```python
from build123d import *

# Parameters (mm, degrees)
CROQUIS1_R              = 1.25
SALIENTE_EXTRUIR3_DEPTH = 3
CROQUIS7_W              = 0.5
CROQUIS7_H              = 4.35
SALIENTE_EXTRUIR4_DEPTH = 1.5
CROQUIS8_R              = 0.75
CORTAR_EXTRUIR1_DEPTH   = 21.944510021
SALIENTE_EXTRUIR5_DEPTH = 1.5
CROQUIS10_R             = 0.5
SALIENTE_EXTRUIR6_DEPTH = 2
CORTAR_EXTRUIR2_REACH   = 27.447
CROQUIS11_W             = 3.6
CROQUIS11_H             = 5.5
CROQUIS12_R             = 2.25
SALIENTE_EXTRUIR8_DEPTH = 3.6
CROQUIS13_R             = 1
SALIENTE_EXTRUIR9_DEPTH = 2.1


with BuildPart() as part:
    # Croquis1 → Saliente-Extruir3 (new, symmetric)
    with BuildSketch(Plane.XY):
        with BuildLine():
            Line((-9.25, 5), (-3.39, 5))
            ThreePointArc((-3.39, 5), (-3.319289322, 4.970710678), (-3.29, 4.9))
            Line((-3.29, 4.9), (-3.29, 4.8))
            ThreePointArc((-3.29, 4.8), (-3.202132034, 4.587867966), (-2.99, 4.5))
            Line((-2.99, 4.5), (9.25, 4.5))
            ThreePointArc((9.25, 4.5), (9.780330086, 4.280330086), (10, 3.75))
            Line((10, 3.75), (10, -4.25))
            ThreePointArc((10, -4.25), (9.780330086, -4.780330086), (9.25, -5))
            Line((9.25, -5), (-9.25, -5))
            ThreePointArc((-9.25, -5), (-9.780330086, -4.780330086), (-10, -4.25))
            Line((-10, -4.25), (-10, 4.25))
            ThreePointArc((-10, 4.25), (-9.780330086, 4.780330086), (-9.25, 5))
        make_face()
        with Locations((-4.5, -2.5)):
            Circle(CROQUIS1_R, mode=Mode.SUBTRACT)
        with Locations((5, -2.5)):
            Circle(CROQUIS1_R, mode=Mode.SUBTRACT)
    extrude(amount=SALIENTE_EXTRUIR3_DEPTH, both=True)

    # Croquis7 → Saliente-Extruir4 (add, symmetric)
    with BuildSketch(Plane.XY):
        with Locations((-8.05, -7.175)):
            Rectangle(CROQUIS7_W, CROQUIS7_H)
        with Locations((0.95, -7.175)):
            Rectangle(CROQUIS7_W, CROQUIS7_H)
        with Locations((8.25, -7.175)):
            Rectangle(CROQUIS7_W, CROQUIS7_H)
    extrude(amount=SALIENTE_EXTRUIR4_DEPTH, both=True)

    # Croquis8 → Cortar-Extruir1 (cut, through all)
    with BuildSketch(Plane(origin=(8.5, 0, 0), x_dir=(0, 0, -1), z_dir=(1, 0, 0))):
        with Locations((0, -7.85)):
            Circle(CROQUIS8_R)
        Polygon((-1.5, -9.152010101), (-1.5, -9.35), (-1.302010101, -9.35), align=None)
        Polygon((1.302010101, -9.35), (1.5, -9.152010101), (1.5, -9.35), align=None)
    extrude(amount=-CORTAR_EXTRUIR1_DEPTH, mode=Mode.SUBTRACT)

    # Croquis9 → Saliente-Extruir5 (add, symmetric)
    with BuildSketch(Plane.XY):
        with BuildLine():
            Line((-1.48, 4.5), (0.52, 4.5))
            Line((0.52, 4.5), (0.52, 6.15))
            ThreePointArc((0.52, 6.15), (0.490710678, 6.220710678), (0.42, 6.25))
            Line((0.42, 6.25), (-1.38, 6.25))
            ThreePointArc((-1.38, 6.25), (-1.450710678, 6.220710678), (-1.48, 6.15))
            Line((-1.48, 6.15), (-1.48, 4.5))
        make_face()
    extrude(amount=SALIENTE_EXTRUIR5_DEPTH, both=True)

    # Croquis10 → Saliente-Extruir6 (add, symmetric)
    with BuildSketch(Plane.XY):
        with BuildLine():
            Line((-6.45, 5), (-6.24, 5))
            ThreePointArc((-6.24, 5), (-6.120788655, 5.324037035), (-5.82, 5.493558507))
            Line((-5.82, 5.493558507), (11.429810709, 8.44212265))
            Line((11.429810709, 8.44212265), (10.840097881, 11.892084791))
            ThreePointArc((10.840097881, 11.892084791), (8.877970038, 13.281348744), (7.488706086, 11.319220901))
            Line((7.488706086, 11.319220901), (8.044721038, 8.066399453))
            Line((8.044721038, 8.066399453), (-6.05083857, 5.657001325))
            ThreePointArc((-6.05083857, 5.657001325), (-6.380057775, 5.449678442), (-6.460998376, 5.06913057))
            Line((-6.460998376, 5.06913057), (-6.45, 5))
        make_face()
        with Locations((9.164401983, 11.605652846)):
            Circle(CROQUIS10_R, mode=Mode.SUBTRACT)
    extrude(amount=SALIENTE_EXTRUIR6_DEPTH, both=True)

    # Croquis11 → Cortar-Extruir2 (cut, up to next)
    with BuildSketch(Plane(origin=(12.50740608, 2.137930074, 0), x_dir=(0, 0, -1), z_dir=(0.9857034690888546, 0.16848937956499643, 0)), mode=Mode.PRIVATE) as cortar_extruir2_sk1:
        with Locations((0, 9.345627867)):
            Rectangle(CROQUIS11_W, CROQUIS11_H)
    cortar_extruir2_tool1 = extrude(cortar_extruir2_sk1.sketch, amount=-CORTAR_EXTRUIR2_REACH, mode=Mode.PRIVATE) & part.part
    add(cortar_extruir2_tool1.solids().sort_by_distance((10.932767, 11.349948, 0))[0], mode=Mode.SUBTRACT)

    # Croquis12 → Saliente-Extruir8 (add)
    with BuildSketch(Plane(origin=(0, 0, 1.8), x_dir=(-1, 0, 0), z_dir=(0, 0, -1))):
        with Locations(Location((-9.164401983, 11.605652846, 0), (0, 0, 211.22606331))):
            Circle(CROQUIS12_R)
    extrude(amount=SALIENTE_EXTRUIR8_DEPTH)

    # Croquis13 → Saliente-Extruir9 (add, symmetric)
    with BuildSketch(Plane.XY):
        with Locations((9.164401983, 11.605652846)):
            Circle(CROQUIS13_R)
    extrude(amount=SALIENTE_EXTRUIR9_DEPTH, both=True)


solid = part.part
```
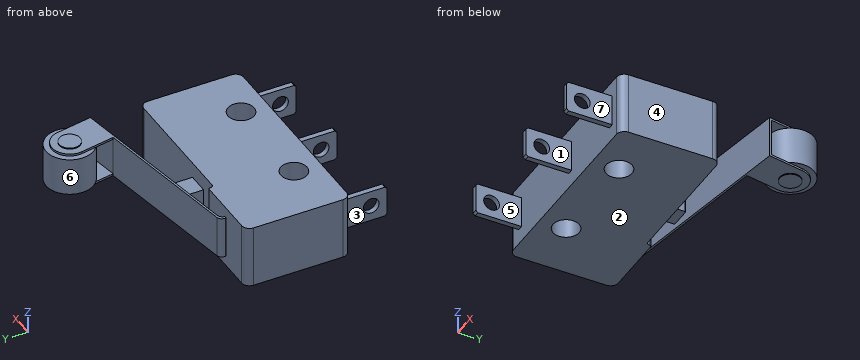
Can you work these out from the model? Positions are in its coordinate system, mm. Face numbers are marked on the shaded views. A direction names the side the tool comes from. Give positions to 0.01 mm unless a question says otherwise; leave off trailing zeros. Loops run counter-clockwise (first coordinate to the right, second up) from the corner with the lowest first, then second, coordinate; pieces in that order, holes last. Notation, with made-up numbers: M 36.25,-34.5 L 44.25,-34.5 A18 cw 44.25,-10.5 Z; hole C 70.5,54.5 d8. An arc over 180 degrees is marked long. One line per item, written item: value.
(1) Suppose I cut it at C-C on x = 5. List the corners of the cut face in (y, z) for me, plus the area to 3 significant figures.
Returned:
outline: M -5,-3 L -3.75,-3 L -3.75,3 L -5,3 Z; M -1.25,-3 L 4.5,-3 L 4.5,3 L -1.25,3 Z; M 7.34,-2 L 7.55,-2 L 7.55,2 L 7.34,2 Z
area: 42.8 mm^2
(2) Will these pins go through, and if not, where does the flat tip stop? pin 1 (2 mm diameter, centred on x = 2, z = 1, fed in from +Y); pin 2 (1.2 mm diameter, centred on x = 10.5, y = 9, fed in from +Z); pin 3 (3.5 mm diameter, centred on y = -7, z = 0, fed in from +X); pin 4 (1.4 mm diameter, centred on x = -0.5, y = 5, fed in from -Z).
Returned:
pin 1: y = 7.2
pin 2: z = 2
pin 3: x = 8.5
pin 4: z = -3
(3) Suppose I cut it at B-B on y = -2.5. List the corners of the cut face in (x, z) for me.
Returned:
outline: M -10,-3 L -5.75,-3 L -5.75,3 L -10,3 Z; M -3.25,-3 L 3.75,-3 L 3.75,3 L -3.25,3 Z; M 6.25,-3 L 10,-3 L 10,3 L 6.25,3 Z
(4) Which directions (+Z, -Z, +X, -X, +Y, -Y) give clear straight access to the entire face, cutting with the end or side of a thin tool? Please do the marked faces 1, 2, 3 and 4.
Returned:
face 1: +Z, -Z, -Y
face 2: -Z, +X, -X, +Y, -Y
face 3: +Z, -Z, -X, -Y
face 4: +Z, -Z, +X, -Y
(5) We'd pull the mould along X, two halves only. Please class the marked faces 5, 6 and 7: released by +X, released by -X, zero draft, split by the parting line, or undercut.
Returned:
face 5: undercut
face 6: split by the parting line
face 7: released by +X
(6) Suppose I cut it at A-A on y = -7.85. List the corners of the cut face in (x, z) for me.
Returned:
outline: M -8.3,-1.5 L -7.8,-1.5 L -7.8,-0.75 L -8.3,-0.75 Z; M -8.3,0.75 L -7.8,0.75 L -7.8,1.5 L -8.3,1.5 Z; M 0.7,-1.5 L 1.2,-1.5 L 1.2,-0.75 L 0.7,-0.75 Z; M 0.7,0.75 L 1.2,0.75 L 1.2,1.5 L 0.7,1.5 Z; M 8,-1.5 L 8.5,-1.5 L 8.5,-0.75 L 8,-0.75 Z; M 8,0.75 L 8.5,0.75 L 8.5,1.5 L 8,1.5 Z
(7) Suppose I cut it at D-D on z = 2.6. List the corners of the cut face in (x, y) for me, plus the area to 3 significant figures.
Returned:
outline: M -10,-4.25 A0.75 ccw -9.25,-5 L 9.25,-5 A0.75 ccw 10,-4.25 L 10,3.75 A0.75 ccw 9.25,4.5 L -2.99,4.5 A0.3 cw -3.29,4.8 L -3.29,4.9 A0.1 ccw -3.39,5 L -9.25,5 A0.75 ccw -10,4.25 Z; hole C -4.5,-2.5 d2.5; hole C 5,-2.5 d2.5
area: 183 mm^2
(8) I need wall thicknesses on line 1 (X direction, y = -6, z = 0.8); line 2 (Y direction, x = -4.5, z = -1); line 3 (Y direction, x = -8.2, z = 0). Which ranges of each line are inside material? Lowest first, please.
Returned:
line 1: -8.3 to -7.8, 0.7 to 1.2, 8 to 8.5
line 2: -5 to -3.75, -1.25 to 5, 5.72 to 5.92
line 3: -9.35 to -8.6, -7.1 to 5
